Study the drawing (mm; zero at the part's minimum x, y, z) and answer. A direction names the side the tool comes from. Give positions to 0.01 mm unless a question says otherwise; leave off trailing zeros. Write each loop counter-clockwise with the first axis right and the second up, starting at its lowest first coordinate (ties: lowest second). Pieces come first, ordered by that corner, then holes. Notation, with made-up numbers: M 32,51.5 L 48,51.5 A31 cw 48,82.5 Z; hole C -33.75,65 d2. An arc over 180 degrees is marked long. Use a Markdown table: item, result. Add a question column.
Item 1: For the marked faces 4 and 5, determine the directions among +Z, -Z, +X, -X, +Y, -Y from which every point of the face is accessible in a straight line to the end or side of a thin tool.
Item 2: A cutting plane is placed at C-C on z = 19.5. Determine the outline of the cut face in (x, y), then the cut area to 3 significant figures.
Item 3: A cutting plane is placed at B-B on y = 44. Determine the outline of the cut face in (x, z).
Item 4: A cutting plane is placed at D-D on x = 34. Determine the outline of the cut face in (y, z).
Item 5: Consider probe 1 along X at (y, z) = (22.5, 46); probe 2 along Y at (x, z) = (27, 24) (1 decimal); probe 3 along Z at (x, y) = (6, 67) (1 decimal). Determine where each line is inside the solid, lowest interval first. Write a range as [from, to].
Item 6: The mould has two halves that part along X. Classify the marked faces 1, 2 and 3: pulls with the +X half, pulls with the -X half, needs draft (parallel to the pull), parting line crosses it, or undercut.
Item 7: Given P1, Ø1, axis at x = 29.5, z = 49.5, coming from the +Y side; P2, Ø5, axis at y = 50, z = 45, coming from the +X side; P3, Ø8, axis at x = 28, z = 20, coming from the +Y side (1 decimal), each flat-ended and moving along its own axis, determine where each tip first touches the part or whether it passes through.
Item 8: A cutting plane is placed at A-A on x = 17.5. Determine the outline of the cut face in (y, z), then the cut area to 3 significant figures.
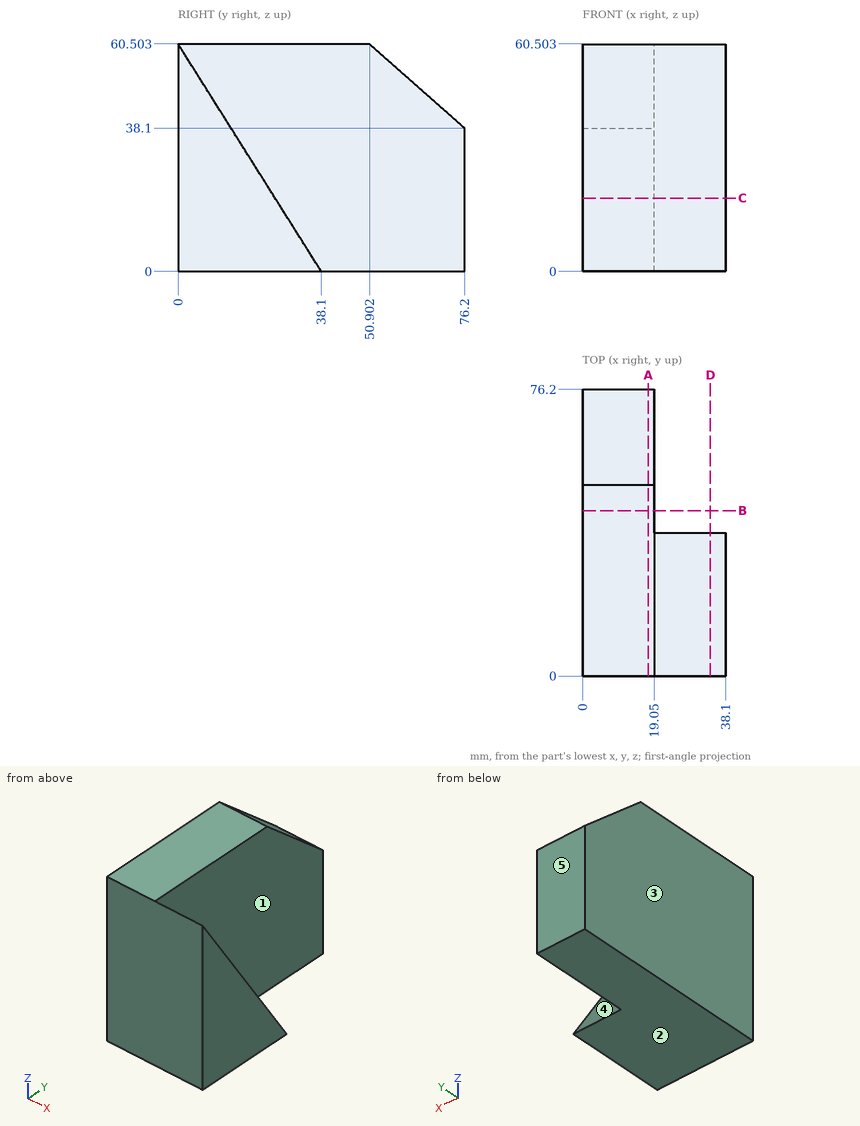
Filled in:
| question | item | result |
|---|---|---|
| 1 | face 4 | +Z, +X, +Y |
| 1 | face 5 | +Z, -Z, +X, -X, +Y |
| 2 | outline | M 0,0 L 38.1,0 L 38.1,25.82 L 19.05,25.82 L 19.05,76.2 L 0,76.2 Z |
| 2 | area | 1,940 mm² |
| 3 | outline | M 0,0 L 19.05,0 L 19.05,60.5 L 0,60.5 Z |
| 4 | outline | M 0,0 L 38.1,0 L 0,60.5 Z |
| 5 | probe 1 | [0, 19.05] |
| 5 | probe 2 | [0, 23] |
| 5 | probe 3 | [0, 46.2] |
| 6 | face 1 | pulls with the +X half |
| 6 | face 2 | needs draft |
| 6 | face 3 | pulls with the -X half |
| 7 | P1 | y = 7.24 |
| 7 | P2 | x = 19.05 |
| 7 | P3 | y = 28 |
| 8 | outline | M 0,0 L 76.2,0 L 76.2,38.1 L 50.9,60.5 L 0,60.5 Z |
| 8 | area | 4,330 mm² |
